```python
from build123d import *

# Parameters (mm, degrees)
SKETCH_R     = 1.8
PAD_DEPTH    = 2
CHAMFER_SIZE = 0.4


with BuildPart() as part:
    # Sketch → Pad (new body)
    with BuildSketch(Plane.XY):
        with BuildLine():
            Line((11, 0), (11, 1))
            ThreePointArc((11, 1), (10.197651, 4.626718), (7.940355, 7.576543))
            Line((1.5, 13), (7.940355, 7.576543))
            Line((1.5, 105), (1.5, 13))
            Line((-1.5, 105), (1.5, 105))
            Line((-1.5, 13), (-1.5, 105))
            Line((-1.5, 13), (-7.940355, 7.576543))
            ThreePointArc((-7.940355, 7.576543), (-10.197651, 4.626718), (-11, 1))
            Line((-11, 1), (-11, 0))
            ThreePointArc((-11, 0), (-9.535534, -3.535534), (-6, -5))
            Line((-6, -5), (6, -5))
            ThreePointArc((6, -5), (9.535534, -3.535534), (11, 0))
        make_face()
        with Locations((-6, 0)):
            Circle(SKETCH_R, mode=Mode.SUBTRACT)
        with Locations((6, 0)):
            Circle(SKETCH_R, mode=Mode.SUBTRACT)
    extrude(amount=PAD_DEPTH)

    # Chamfer
    chamfer_edges = [part.edges().sort_by_distance(p)[0] for p in [
        (-7.8, 0, 2),
        (4.2, 0, 2),
    ]]
    chamfer(chamfer_edges, length=CHAMFER_SIZE)


solid = part.part
```
Here's how the part is built. I have some questions about the finished solid (model axes, mm). A direction names the side the tool comes from. Coordinates: 2 decimals unless noted, no trailing zeros. Order: outer loops, then holes, each group sorted by start corner. A loop starts at its lowest first (then second) coordinate and runs counter-clockwise, first axis right, second up. Notation, with made-up numbers: (68.25, -34) -> (98.25, -34) arc R15 ccw to (98.25, -21) -> close; hole circle Ø6 at (-20.5, -6.75). An arc over 180 degrees is marked (long way). Return JSON: item names as keys, results as strings.
1) If we section it at B-B on y = 27.5: List the corners of the cut face in (x, z) for me.
Conclusion:
{"outline": "(-1.5, 0) -> (1.5, 0) -> (1.5, 2) -> (-1.5, 2) -> close"}
2) If I drill on probe 1 along Y at (x, z) = (-6, 1.35); probe 2 along Y at (x, z) = (7, 0.4); probe 3 along X at (y, z) = (69.5, 1.1), over which ranges is the centre line in solid material (lowest first)?
Conclusion:
{"probe 1": "y = -5 to -1.8, 1.8 to 9.21", "probe 2": "y = -4.9 to -1.5, 1.5 to 8.37", "probe 3": "x = -1.5 to 1.5"}
3) I'm going to push a flat-ended pin straight in: P1, Ø0.6, axis at y = 64, z = 1, coming from the -X side. Where does the tip first touch, or does it pass through?
Conclusion:
{"P1": "stops at x = -1.5"}
4) If we section it at A-A on z = 0.55: List the corners of the cut face in (x, y) for me, plus the area to 3 significant figures.
Conclusion:
{"outline": "(-11, 0) arc R5 ccw to (-6, -5) -> (6, -5) arc R5 ccw to (11, 0) -> (11, 1) arc R8.6 ccw to (7.94, 7.58) -> (1.5, 13) -> (1.5, 105) -> (-1.5, 105) -> (-1.5, 13) -> (-7.94, 7.58) arc R8.6 ccw to (-11, 1) -> close; hole circle Ø3.6 at (-6, 0); hole circle Ø3.6 at (6, 0)", "area": "561 mm²"}
5) On a 3-axis mill with a long thin cutter (end or side, diameter ignored), from which of +Z, -Z, +X, -X, +Y, -Y can I reach the whole of each face in a straight line? I mean faces 5 (the flat face through (-1.5, 58, 1)), 6 (the flat face through (0, 26, 0)). Say none if no direction works.
Conclusion:
{"face 5": "+Z, -Z, -X, +Y", "face 6": "-Z, +X, -X, +Y, -Y"}
6) Thinking about a two-plate mould opening in X: for faces 1 (the cylindrical face through (-4.283, 0.541, 0.789)), 2 (the flat face through (0, 26, 2)), 3 (the cylindrical face through (7.717, 0.541, 0.789)), 4 (the flat face through (1.5, 60, 1)), which applies, +X half, -X half, draft (parallel to the pull), parting line (faces both ways), or undercut?
Conclusion:
{"face 1": "undercut", "face 2": "draft", "face 3": "undercut", "face 4": "+X half"}
